Geometry check sheet. Reference: the model listing, model coordinates, mm. Give positions to 0.01 mm unless a question says otherwise; leave off trailing zeros. Order: outer loops, then holes, each group sorted by start corner. A loop starts at its lowest first (then second) coordinate and runs counter-clockwise, first axis right, second up. Notation, with made-up numbers: M 64.5,26.25 L 93.5,26.25 A21 cw 93.5,56.25 Z; hole C 18.25,18.25 d4. An arc over 180 degrees is marked long. Answer as CSV lines item,"result". Start each with the question number.
```python
from build123d import *

# Parameters (mm, degrees)
SKETCH_1_W          = 150
SKETCH_1_H          = 150
EXTRUDE_1_DEPTH     = 3
SKETCH_4_R          = 2.55
SKETCH_4_R_2        = 3.5
CUT_EXTRUDE_3_DEPTH = 7
FILLET_1_R          = 8
SKETCH_6_W          = 70
SKETCH_6_H          = 60
SKETCH_6_R          = 2.55
EXTRUDE_2_DEPTH     = 3
FILLET_2_R          = 20
FILLET_3_R          = 15
SKETCH_7_R          = 1.6
CUT_EXTRUDE_5_DEPTH = 10


with BuildPart() as part:
    # 草图1 → 凸台-拉伸1 (new body)
    with BuildSketch(Plane.XY):
        Rectangle(SKETCH_1_W, SKETCH_1_H)
    extrude(amount=EXTRUDE_1_DEPTH)

    # 草图4 → 切除-拉伸3 (cut)
    with BuildSketch(Plane.XY.offset(3)):
        with Locations((-67, 67)):
            Circle(SKETCH_4_R)
        with Locations((-67, -67)):
            Circle(SKETCH_4_R)
        with Locations((67, -67)):
            Circle(SKETCH_4_R)
        with Locations((67, 67)):
            Circle(SKETCH_4_R)
        Circle(SKETCH_4_R_2)
    extrude(amount=-CUT_EXTRUDE_3_DEPTH, mode=Mode.SUBTRACT)

    # 圆角1
    fillet_1_edges = [part.edges().sort_by_distance(p)[0] for p in [
        (75, -75, 1.5),
        (-75, -75, 1.5),
        (-75, 75, 1.5),
        (75, 75, 1.5),
    ]]
    fillet(fillet_1_edges, radius=FILLET_1_R)

    # 草图6 → 凸台-拉伸2 (add)
    with BuildSketch(Plane.XY.offset(3)):
        with Locations((-110, 0)):
            Rectangle(SKETCH_6_W, SKETCH_6_H)
        with Locations((-125, 0)):
            Circle(SKETCH_6_R, mode=Mode.SUBTRACT)
    extrude_2 = extrude(amount=-EXTRUDE_2_DEPTH)

    # 镜向1: 凸台-拉伸2 across plane
    add(extrude_2.mirror(Plane(origin=(0, 0, 0), x_dir=(0, 0, 1), z_dir=(1, 0, 0))))

    # 圆角2
    fillet_2_edges = [part.edges().sort_by_distance(p)[0] for p in [
        (-75, -30, 1.5),
        (-75, 30, 1.5),
        (75, -30, 1.5),
        (75, 30, 1.5),
    ]]
    fillet(fillet_2_edges, radius=FILLET_2_R)

    # 圆角3
    fillet_3_edges = [part.edges().sort_by_distance(p)[0] for p in [
        (-145, 30, 1.5),
        (-145, -30, 1.5),
        (145, 30, 1.5),
        (145, -30, 1.5),
    ]]
    fillet(fillet_3_edges, radius=FILLET_3_R)

    # 草图7 → 切除-拉伸5 (cut)
    with BuildSketch(Plane.XY.offset(3)):
        with Locations((0, 42.5)):
            Circle(SKETCH_7_R)
        with Locations((0, -42.5)):
            Circle(SKETCH_7_R)
    extrude(amount=-CUT_EXTRUDE_5_DEPTH, mode=Mode.SUBTRACT)


solid = part.part
```
Item 1: Draft check along Y on faces 1 (the face through (122.57, 0.77, 1.52)), 2 (the face through (-2, -16, 0)), 3 (the face through (3.233, -1.341, 1.521)), 4 (the face through (140.72, 25.49, 1.48)). Enter one of: pulls with the +Y half, pulls with the -Y half, needs draft (parallel to the pull), parting line crosses it, or undercut.
Item 2: Section check A-A on z = 2. Give the number of separate pieces and of enclosed holes in the cut face, then the cut area to 3 significant figures.
Item 3: Section check B-B on y = 55. Record the boundary of the cut face in (x, z).
Item 4: Depth check by flat-ended pin: pin 1 Ø8 at (x, y) = (0, 0) entering from -Z; pin 2 Ø4 at (x, y) = (-125, 0) entering from -Z (1 decimal); pin 3 Ø0.9 at (x, z) = (110.5, 2) entering from +Y; pin 4 Ø1.5 at (y, z) = (-56.5, 1) entering from +X. Enter the tip coordinate at first touch or a pass-through.
Item 5: Scan lines: line 1 along Y through (x, z) = (67, 2.3); line 2 along Y through (x, z) = (0, 1.3); line 3 along X through (y, z) = (53.5, 0.5). Record each from-to range of solid material in increasing order.
Numbers:
1,face 1,"undercut"
1,face 2,"needs draft"
1,face 3,"undercut"
1,face 4,"pulls with the +Y half"
2,separate pieces,"1"
2,enclosed holes,"9"
2,area,"30,800 mm2"
3,outline,"M -75,0 L 75,0 L 75,3 L -75,3 Z"
4,pin 1,"z = 0"
4,pin 2,"through"
4,pin 3,"y = 30"
4,pin 4,"x = 75"
5,line 1,"-75 to -69.55, -64.45 to 64.45, 69.55 to 75"
5,line 2,"-75 to -44.1, -40.9 to -3.5, 3.5 to 40.9, 44.1 to 75"
5,line 3,"-75 to 75"
